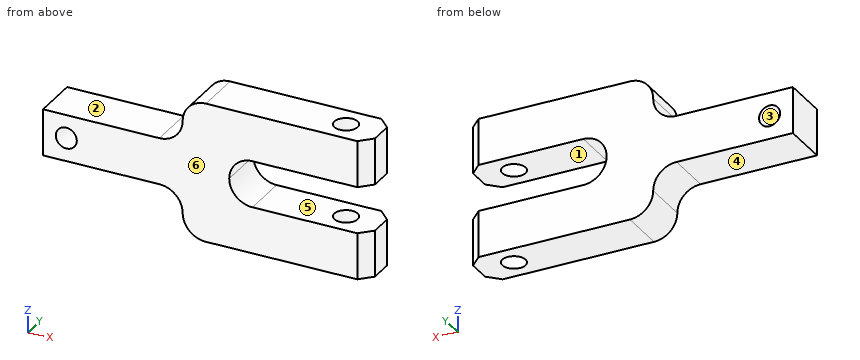
from build123d import *

# Parameters (mm, degrees)
F0_R     = 5.7374218315
F1_DEPTH = 12.7
F2_R     = 12.69999
F3_R     = 12.69999
F4_R     = 12.69999
F5_SIZE2 = 6.35
F5_SIZE  = 6.35
F6_SIZE2 = 6.35
F6_SIZE  = 6.35
F7_R     = 6.35
F8_DEPTH = 127


# Not quite as in the source:
# - a fillet or chamfer is up to 0.001 mm smaller than in the source, because OpenCascade refuses the exact size


with BuildPart() as f1:
    # F0 (on Front) → F1 (new body, symmetric)
    with BuildSketch(Plane.XZ):
        Polygon((26.8901219662, -12.7), (26.8901219662, 12.7), (1.4901219662, 12.7), (-74.7098780338, 12.7), (-74.7098780338, -12.7), (1.4901219662, -12.7), align=None)
        with Locations((-62.0098780338, 0)):
            Circle(F0_R, mode=Mode.SUBTRACT)
        Polygon((1.4901219662, 12.7), (26.8901219662, 12.7), (103.0901219662, 12.7), (103.0901219662, 38.1), (1.4901219662, 38.1), align=None)
        Polygon((103.0901219662, -12.7), (26.8901219662, -12.7), (1.4901219662, -12.7), (1.4901219662, -38.1), (103.0901219662, -38.1), align=None)
    extrude(amount=F1_DEPTH, both=True)

    # F2 (radius 12.7 in the source; OpenCascade refuses exactly that, so slightly less here)
    f2_edges = [f1.edges().sort_by_distance(p)[0] for p in [
        (1.490122, 0, 38.1),
        (1.490122, 0, 12.7),
    ]]
    fillet(f2_edges, radius=F2_R)

    # F3 (radius 12.7 in the source; OpenCascade refuses exactly that, so slightly less here)
    f3_edges = [f1.edges().sort_by_distance(p)[0] for p in [
        (26.890122, 0, 12.7),
        (26.890122, 0, -12.7),
    ]]
    fillet(f3_edges, radius=F3_R)

    # F4 (radius 12.7 in the source; OpenCascade refuses exactly that, so slightly less here)
    f4_edges = [f1.edges().sort_by_distance(p)[0] for p in [
        (1.490122, 0, -12.7),
        (1.490122, 0, -38.1),
    ]]
    fillet(f4_edges, radius=F4_R)

    # F5
    f5_edges = [f1.edges().sort_by_distance(p)[0] for p in [
        (103.090122, -12.7, 25.4),
        (103.090122, 12.7, 25.4),
    ]]
    chamfer(f5_edges, length=F5_SIZE, length2=F5_SIZE2)

    # F6
    f6_edges = [f1.edges().sort_by_distance(p)[0] for p in [
        (103.090122, -12.7, -25.4),
        (103.090122, 12.7, -25.4),
    ]]
    chamfer(f6_edges, length=F6_SIZE, length2=F6_SIZE2)

    # F7 (on Top) → F8 (cut, symmetric)
    with BuildSketch(Plane.XY):
        with Locations((84.0401219662, 0)):
            Circle(F7_R)
    extrude(amount=F8_DEPTH, both=True, mode=Mode.SUBTRACT)


solid = f1.part
For this review, take the finished solid that the model builds, in its own axes (mm). Face numbers are marked on the shaded views. A direction names the side the tool comes from. Round coordinates to 2 decimals unless told otherwise and drop trailing zeros. Order: outer loops, then holes, each group sorted by start corner. A loop starts at its lowest first (then second) coordinate and runs counter-clockwise, first axis right, second up. Notation, with made-up numbers: (41, 80.5) -> (71, 80.5) arc R21 cw to (71, 113.5) -> close; hole circle Ø9 at (-22, -28). An arc over 180 degrees is marked (long way). Write item = value, one per line. Start each with the question number.
1) Take a section at D-D on z = -31. State the section outline as (x, y) points.
2) Take a section at C-C on x = 62. State the section outline as (y, z) points, plus the area to 3 significant figures.
3) The part is to be moulded in two halves that separate along Z. For the marked faces 4, 5 and 6, say which applies: +Z half, -Z half, draft (parallel to the pull), parting line (faces both ways), or undercut.
4) Take a section at A-A on y = 0. Count the separate pieces of the cut face and the enclosed holes in it, plus the area to 3 significant figures.
5) Insertion check: pin 1 (7.5 mm diameter, centred on x = -32.5, y = -1, fed in from +Z). The pin has a flat end and moves straight along its axis. Give the tip position at first contact, or say it passes through.
6) Tool access review of the marked faces 1, 2 and 3: name each direction out of +Z, -Z, +X, -X, +Y, -Y from which nothing blocks a thin tool from reaching the whole face with its end or side.
7) Take a section at B-B on x = 83. State the section outline as (y, z) points.
8) To check wall thickness, follow line 1 (Z direction, x = 74.5, y = -0.5); line 2 (Z direction, x = 38, y = 5.5); line 3 (X direction, y = 7, z = -3.5). State the ranges of each line that lie inside material, in increasing order. Write a range as from..to.
Verdict:
q1.outline = (2.79, -12.7) -> (96.74, -12.7) -> (103.09, -6.35) -> (103.09, 6.35) -> (96.74, 12.7) -> (2.79, 12.7) -> close; hole circle Ø12.7 at (84.04, 0)
q2.outline = (-12.7, -38.1) -> (12.7, -38.1) -> (12.7, -12.7) -> (-12.7, -12.7) -> close; (-12.7, 12.7) -> (12.7, 12.7) -> (12.7, 38.1) -> (-12.7, 38.1) -> close
q2.area = 1,290 mm2
q3.face_4 = -Z half
q3.face_5 = undercut
q3.face_6 = draft
q4.separate_pieces = 3
q4.enclosed_holes = 1
q4.area = 7,060 mm2
q5.pin_1 = 12.7
q6.face_1 = +X, +Y, -Y
q6.face_2 = +Z, -X, +Y, -Y
q6.face_3 = +Y, -Y
q7.outline = (-12.7, -38.1) -> (-6.26, -38.1) -> (-6.26, -12.7) -> (-12.7, -12.7) -> close; (-12.7, 12.7) -> (-6.26, 12.7) -> (-6.26, 38.1) -> (-12.7, 38.1) -> close; (6.26, -38.1) -> (12.7, -38.1) -> (12.7, -12.7) -> (6.26, -12.7) -> close; (6.26, 12.7) -> (12.7, 12.7) -> (12.7, 38.1) -> (6.26, 38.1) -> close
q8.line_1 = -38.1..-12.7, 12.7..38.1
q8.line_2 = -38.1..-12.6, 12.6..38.1
q8.line_3 = -74.71..-66.56, -57.46..27.38
